The listing builds one solid part. Answer for the finished solid, in the listing's coordinates (mm). Face numbers are marked on the shaded views. A direction names the side the tool comes from. Round coordinates to 2 decimals unless told otherwise and drop trailing zeros. Write each loop counter-clockwise with the first axis right and the second up, starting at its lowest first coordinate (ties: lowest second). Pieces come first, ordered by that corner, then holes. Notation, with made-up numbers: (40, 79) - (65, 79) arc R23 ccw to (65, 94) - close; hole circle Ø8 at (1, 11.5). An arc over 180 degrees is marked (long way). Use a Markdown table: item, result. Add a question column.
1) A tool of negligible diameter and unlimited length cuts with its end or side. For the marked faces 1 and 2, from which of +Z, -Z, +X, -X, +Y, -Y can it reach the whole face along a straight path? Write none if from no direction.
2) A cutting plane is placed at B-B (y = 51). Give the vertices of the cut face in (x, z).
3) Each of these flat-tipped pins is pushed along its axis until it touches: P1, Ø9, axis at y = 0, z = -8, coming from the +X side; P2, Ø4.5, axis at x = 189, y = -3.5, coming from the -Z side; P3, Ø12.5, axis at x = -175.5, z = -7, coming from the +Y side. Where does it stop, or does it pass through?
4) A cutting plane is placed at D-D (y = 85). Give the vertices of the cut face in (x, z), then the cut area to 3 significant figures.
5) A cutting plane is placed at A-A (x = 169.5). Give the vertices of the cut face in (y, z), then the cut area to 3 significant figures.
6) Find the intervals of material crossed by probe 1 along X at (y, z) = (24.5, 36); probe 2 along Y at (x, z) = (4, 35); probe 3 along X at (y, z) = (90, 3), in increasing order. Write a range as from..to.
7) Determine the mould class of the marked faces 3, 4 and 5 for opening direction X: +X half, -X half, draft (parallel to the pull), parting line (faces both ways), or undercut.
8) A cutting plane is placed at C-C (z = 12.5). Give the vertices of the cut face in (x, y).
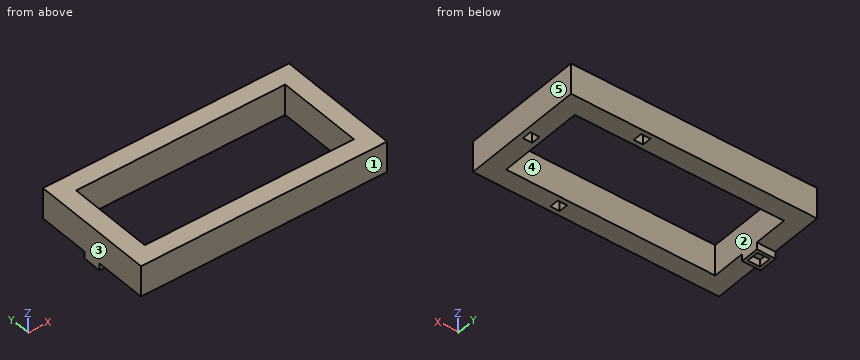
```python
from build123d import *

# Parameters (mm, degrees)
SKETCH1_W           = 400
SKETCH1_H           = 200
SKETCH1_W_2         = 340
SKETCH1_H_2         = 140
BOSS_EXTRUDE1_DEPTH = 50
SKETCH2_W           = 15
SKETCH2_H           = 15
CUT_EXTRUDE1_DEPTH  = 40
SKETCH3_W           = 30
SKETCH3_H           = 30
SKETCH3_W_2         = 20
SKETCH3_H_2         = 20
BOSS_EXTRUDE2_DEPTH = 11.5


with BuildPart() as part:
    # Sketch1 → Boss-Extrude1 (new body)
    with BuildSketch(Plane.XY):
        with Locations((5.416666667, 0)):
            Rectangle(SKETCH1_W, SKETCH1_H)
        with Locations((5.416666667, 0)):
            Rectangle(SKETCH1_W_2, SKETCH1_H_2, mode=Mode.SUBTRACT)
    extrude(amount=BOSS_EXTRUDE1_DEPTH)

    # Sketch2 → Cut-Extrude1 (cut)
    with BuildSketch(Plane(origin=(0, 0, 0), x_dir=(-1, 0, 0), z_dir=(0, 0, -1))):
        with Locations((-77.916666667, 85)):
            Rectangle(SKETCH2_W, SKETCH2_H)
        with Locations((-77.916666667, -85)):
            Rectangle(SKETCH2_W, SKETCH2_H)
        Polygon((-197.916664047, 7.493396785), (-197.916664047, -7.506603215), (-182.916666667, -7.497737374), (-182.916666667, 7.502262626), align=None)
    extrude(amount=-CUT_EXTRUDE1_DEPTH, mode=Mode.SUBTRACT)

    # Sketch3 → Boss-Extrude2 (add)
    with BuildSketch(Plane(origin=(0, 0, 0), x_dir=(-1, 0, 0), z_dir=(0, 0, -1))):
        with Locations((179.583333333, 0)):
            Rectangle(SKETCH3_W, SKETCH3_H)
        with Locations((179.583333333, 0)):
            Rectangle(SKETCH3_W_2, SKETCH3_H_2, mode=Mode.SUBTRACT)
    extrude(amount=BOSS_EXTRUDE2_DEPTH)


solid = part.part
```
Entries:
| question | item | result |
|---|---|---|
| 1 | face 1 | +Z, -Z, +X, -X, -Y |
| 1 | face 2 | +Z, -Z |
| 2 | outline | (-194.58, 0) - (-164.58, 0) - (-164.58, 50) - (-194.58, 50) - close; (175.42, 0) - (205.42, 0) - (205.42, 50) - (175.42, 50) - close |
| 3 | P1 | stops at x = -164.58 |
| 3 | P2 | stops at z = 40 |
| 3 | P3 | stops at y = 15 |
| 4 | outline | (-194.58, 0) - (70.42, 0) - (70.42, 40) - (85.42, 40) - (85.42, 0) - (205.42, 0) - (205.42, 50) - (-194.58, 50) - close |
| 4 | area | 19,400 mm² |
| 5 | outline | (-100, 0) - (-70, 0) - (-70, 50) - (-100, 50) - close; (70, 0) - (100, 0) - (100, 50) - (70, 50) - close |
| 5 | area | 3,000 mm² |
| 6 | probe 1 | x = -194.58..-164.58, 175.42..205.42 |
| 6 | probe 2 | y = -100..-70, 70..100 |
| 6 | probe 3 | x = -194.58..70.42, 85.42..205.42 |
| 7 | face 3 | -X half |
| 7 | face 4 | undercut |
| 7 | face 5 | +X half |
| 8 | outline | (-194.58, -100) - (205.42, -100) - (205.42, 100) - (-194.58, 100) - close; hole (-164.58, -70) - (175.42, -70) - (175.42, 70) - (-164.58, 70) - close; hole (70.42, -92.5) - (85.42, -92.5) - (85.42, -77.5) - (70.42, -77.5) - close; hole (70.42, 77.5) - (85.42, 77.5) - (85.42, 92.5) - (70.42, 92.5) - close; hole (182.92, -7.5) - (197.92, -7.51) - (197.92, 7.49) - (182.92, 7.5) - close |
